from build123d import *

# Parameters (mm, degrees)
F0_W     = 133.35
F0_H     = 107.95
F1_DEPTH = 76.2
F2_W     = 127
F2_H     = 101.6
F3_DEPTH = 76.2
F4_DEPTH = 73.66
F5_DEPTH = 76.2
F6_T     = -2.5
F7_R     = 40
F8_R     = 4
F9_R     = 5
F10_R    = 40


with BuildPart() as f1:
    # F0 (on Top) → F1 (new body)
    with BuildSketch(Plane.XY):
        Rectangle(F0_W, F0_H)
    extrude(amount=F1_DEPTH)

    # F2 (on Top) → F3 (cut)
    with BuildSketch(Plane.XY):
        Rectangle(F2_W, F2_H)
    extrude(amount=F3_DEPTH, mode=Mode.SUBTRACT)

    # F4 (cut): a face of the model
    f4_faces = [f1.faces().sort_by_distance(p)[0] for p in [
        (64.9593244771, 0, 76.2),
    ]]
    extrude(f4_faces, amount=-F4_DEPTH, mode=Mode.SUBTRACT)

    # F2 (on Top) → F5 (join)
    with BuildSketch(Plane.XY):
        Rectangle(F2_W, F2_H)
    extrude(amount=F5_DEPTH)

    # F6
    f6_openings = [f1.faces().sort_by_distance(p)[0] for p in [
        (0, 0, 0),
    ]]
    offset(amount=F6_T, openings=f6_openings, kind=Kind.INTERSECTION)

    # F7
    f7_edges = [f1.edges().sort_by_distance(p)[0] for p in [
        (-61, 0, 73.7),
        (61, 0, 73.7),
    ]]
    fillet(f7_edges, radius=F7_R)

    # F8
    f8_edges = [f1.edges().sort_by_distance(p)[0] for p in [
        (-49.284271, -48.3, 61.984271),
        (49.284271, 48.3, 61.984271),
    ]]
    fillet(f8_edges, radius=F8_R)

    # F9
    f9_edges = [f1.edges().sort_by_distance(p)[0] for p in [
        (66.675, 53.975, 1.27),
        (66.675, -53.975, 1.27),
        (-66.675, -53.975, 1.27),
        (-66.675, 53.975, 1.27),
    ]]
    fillet(f9_edges, radius=F9_R)

    # F10
    f10_edges = [f1.edges().sort_by_distance(p)[0] for p in [
        (-63.5, 0, 76.2),
        (63.5, 0, 76.2),
    ]]
    fillet(f10_edges, radius=F10_R)


solid = f1.part
Geometry check sheet. Reference: the model listing, model coordinates, mm. A direction names the side the tool comes from. Give positions to 0.01 mm unless a question says otherwise; leave off trailing zeros. Loops run counter-clockwise (first coordinate to the right, second up) from the corner with the lowest first, then second, coordinate; pieces in that order, holes last. Notation, with made-up numbers: (-16, -33.5) -> (-9, -33.5) arc R27 ccw to (-9, 1.5) -> close; hole circle Ø10 at (20, -31). An arc over 180 degrees is marked (long way). Answer in a Markdown table with one row per item. Add a question column.
1) Cross-section at C-C on y = -16. Record the boundary of the cut face in (x, z) (3 decimals).
2) Set-up check for faces 1 (the face through (63.5, -1, 19)), 2 (the face through (-65.25, 52.47, 1.29)), 3 (the face through (61, -1, 17)): record each of +Z, -Z, +X, -X, +Y, -Y from which the full face is reachable in a straight line by a thin tool's end or side.
3) Material ranges on probe 1 along Y at (x, z) = (-46, 57.5); probe 2 along X at (y, z) = (-20.5, 7); probe 3 along X at (y, z) = (-11, 52), recorded low to high. Write a range as from..to.
4) Gauge pin test, flat ends, axial feed: P1, Ø2, axis at x = -22.5, z = 38, coming from the -Y side; P2, Ø8, axis at x = 17.5, y = -13.5, coming from the -Z side; P3, Ø12, axis at x = 39, z = 41.5, coming from the +Y side. Record the tip position at first contact, or that the pin passes through.
5) Draft check along X on faces 4 (the face through (-59.859, -47.097, 17.106)), 5 (the face through (-5, -52, 2.54)), 6 (the face through (-63.5, -1, 19)). Enter one of: pulls with the +X half, pulls with the -X half, needs draft (parallel to the pull), parting line crosses it, or undercut.
6) Cross-section at A-A on x = -19. Record the boundary of the cut face in (y, z) (3 decimals).
7) Cross-section at B-B on z = 31. Record the boundary of the cut face in (x, y), and give its area (3 significant figures).
Outcome:
| question | item | result |
|---|---|---|
| 1 | outline | (-66.675, 0) -> (-64.175, 0) -> (-64.175, 0.04) -> (-61, 0.04) -> (-61, 33.7) arc R40 cw to (-21, 73.7) -> (21, 73.7) arc R40 cw to (61, 33.7) -> (61, 0.04) -> (64.175, 0.04) -> (64.175, 0) -> (66.675, 0) -> (66.675, 2.54) -> (63.5, 2.54) -> (63.5, 36.2) arc R40 ccw to (23.5, 76.2) -> (-23.5, 76.2) arc R40 ccw to (-63.5, 36.2) -> (-63.5, 2.54) -> (-66.675, 2.54) -> close |
| 2 | face 1 | +Z, +X, +Y, -Y |
| 2 | face 2 | +Z, -Z, -X, +Y |
| 2 | face 3 | -Z |
| 3 | probe 1 | y = -50.8..-48.3, 48.3..50.8 |
| 3 | probe 2 | x = -63.5..-61, 61..63.5 |
| 3 | probe 3 | x = -60.25..-56.57, 56.57..60.25 |
| 4 | P1 | stops at y = -50.8 |
| 4 | P2 | stops at z = 73.7 |
| 4 | P3 | stops at y = 50.8 |
| 5 | face 4 | undercut |
| 5 | face 5 | needs draft |
| 5 | face 6 | pulls with the -X half |
| 6 | outline | (-53.975, 0) -> (-51.475, 0) -> (-51.475, 0.04) -> (-48.3, 0.04) -> (-48.3, 69.7) arc R4 cw to (-44.3, 73.7) -> (44.3, 73.7) arc R4 cw to (48.3, 69.7) -> (48.3, 0.04) -> (51.475, 0.04) -> (51.475, 0) -> (53.975, 0) -> (53.975, 2.54) -> (50.8, 2.54) -> (50.8, 76.2) -> (-50.8, 76.2) -> (-50.8, 2.54) -> (-53.975, 2.54) -> close |
| 7 | outline | (-63.5, -50.8) -> (63.5, -50.8) -> (63.5, 50.8) -> (-63.5, 50.8) -> close; hole (-61, -44.3) arc R4 ccw to (-57, -48.3) -> (57, -48.3) arc R4 ccw to (61, -44.3) -> (61, 44.3) arc R4 ccw to (57, 48.3) -> (-57, 48.3) arc R4 ccw to (-61, 44.3) -> close |
| 7 | area | 1,130 mm^2 |
